Can you work these out from the model? Positions are in its coordinate system, mm. A direction names the side the tool comes from. Round coordinates to 2 decimals unless told otherwise and drop trailing zeros. Order: outer loops, then holes, each group sorted by start corner. A loop starts at its lowest first (then second) coordinate and runs counter-clockwise, first axis right, second up.
from build123d import *

# Parameters (mm, degrees)
SFAZOWANIE1_SIZE  = 0.5
SFAZOWANIE1_SIZE2 = 0.288675135


with BuildPart() as part:
    # Szkic1 → Obrót1 (revolve)
    with BuildSketch(Plane.XY):
        Polygon((0, 6), (7, 6), (7, 7), (1, 7), (1, 10), (0, 10), align=None)
    revolve(axis=Axis((0, 0, 0), (1, 0, 0)))

    # Sfazowanie1
    sfazowanie1_edges = [part.edges().sort_by_distance(p)[0] for p in [
        (7, -7, 0),
    ]]
    sfazowanie1_side = [part.faces().sort_by_distance(p)[0] for p in [
        (4, -7, 0),
    ]]
    chamfer(sfazowanie1_edges, length=SFAZOWANIE1_SIZE, length2=SFAZOWANIE1_SIZE2, reference=sfazowanie1_side[0])


solid = part.part
(1) On a 3-axis mill with a long thin cutter (end or side, diameter ignored), from which of +Z, -Z, +X, -X, +Y, -Y can I reach the whole of each face in a straight line? I mean faces 1 (the face through (1, -2, 7)), 2 (the face through (0, 7, 0)). Say none if no direction works.
(2) If we mould it in two halves opening along Y, with no side actions, what happens to faces 3 (the face through (7, 2, -6)), 4 (the face through (3.712, 6.466, -2.681)), 5 (the face through (4, -6, 0))? For each: pulls with the +Y half, pulls with the -Y half, needs draft (parallel to the pull), parting line crosses it, or undercut.
(3) Please list where these lines run through material, in increasing order: probe 1 along Z at (x, y) = (3.5, -0.25); probe 2 along X at (y, z) = (-2, 8.5).
(4) I want a section at B-B, the plane x = 0.5. List the corners of the cut face in (y, z) for me.
(5) I want a section at D-D, the plane x = 4.25. List the corners of the cut face in (y, z) for me.
(6) I'm going to push flat-ended pins straight in: pin 1 Ø2 at (x, z) = (5, 0.5) entering from -Y; pin 2 Ø1.5 at (y, z) = (-8, 0) entering from +X; pin 3 Ø3 at (x, z) = (3.5, -3) entering from +Y. Where does each tip first touch, or does it pass through?
(7) I want a section at C-C, the plane z = -7.5. List the corners of the cut face in (x, y) for me, plus the area to 3 significant figures.
(8) I want a section at A-A, the plane y = 0. List the corners of the cut face in (x, z) for me.
Ans:
1. face 1: +X
1. face 2: +Z, -Z, -X, +Y, -Y
2. face 3: needs draft
2. face 4: parting line crosses it
2. face 5: undercut
3. probe 1: z = -7 to -5.99, 5.99 to 7
3. probe 2: x = 0 to 1
4. outline: circle Ø20 at (0, 0); hole circle Ø12 at (0, 0)
5. outline: circle Ø14 at (0, 0); hole circle Ø12 at (0, 0)
6. pin 1: stops at y = -7
6. pin 2: stops at x = 1
6. pin 3: stops at y = 6.84
7. outline: (0, -6.61) - (1, -6.61) - (1, 6.61) - (0, 6.61) - close
7. area: 13.2 mm2
8. outline: (0, -10) - (1, -10) - (1, -7) - (6.5, -7) - (7, -6.71) - (7, -6) - (0, -6) - close; (0, 6) - (7, 6) - (7, 6.71) - (6.5, 7) - (1, 7) - (1, 10) - (0, 10) - close
